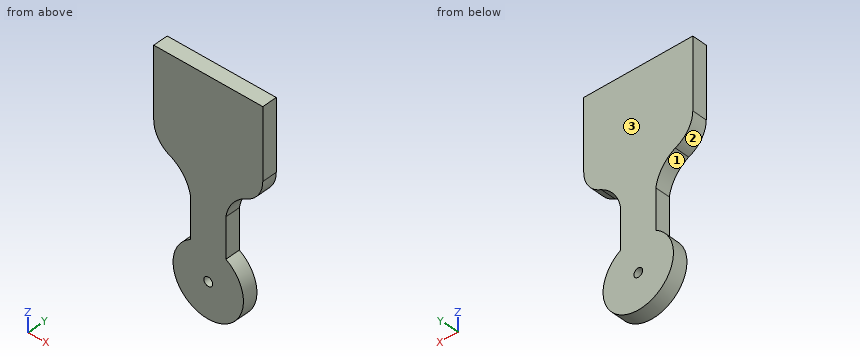
Autodesk Inventor part; units mm, degrees
ref_plane "YZ Plane" through (0, 0, 0) normal (1, 0, 0) x (0, 1, 0)
ref_plane "XZ Plane" through (0, 0, 0) normal (0, 1, 0) x (-1, 0, 0)
ref_plane "XY Plane" through (0, 0, 0) normal (0, 0, 1) x (1, 0, 0)
sketch "Sketch1" plane through (0, 0, 0) normal (0, 1, 0) x (-1, 0, 0)
  line L0 (-5, 10.0042) -> (5, 10.0042)
  line L1 (5, 10.0042) -> (5, -14.9958)
  line L2 (5, -14.9958) -> (-5, -14.9958)
  line L3 (-5, -14.9958) -> (-5, 10.0042)
  circle A0 centre (0, -24.9958) radius 10
  circle A1 centre (0, -24.9958) radius 1.25
  line L4 (-5, -14.9958) -> (-5, -16.3355)
  line L5 (5, -14.9958) -> (5, -16.3355)
  line L6 (-15.5, 30.0042) -> (15.5, 30.0042)
  line L7 (15.5, 30.0042) -> (15.5, 10.0042)
  line L8 (15.5, 10.0042) -> (-15.5, 10.0042)
  line L9 (-15.5, 10.0042) -> (-15.5, 30.0042)
  arc A2 (-5, -5) -> (-10.4985, 2.7374) centre (-15.4294, -6.5891) ccw
  arc A3 (-15.5, 10.0042) -> (-10.4985, 2.7374) centre (-7.7202, 10.0042) ccw
  line L10 (0, 46.7954) -> (0, -49.019) construction
  line L11 (-15.5, 10.0042) -> (-5, 10.0042)
  point P0 (0, 0)
  point P1 (0, -14.9958)
  point P2 (0, 10.0042)
  point P3 (0, 10.0042)
  dimension "d0" = 25
  dimension "d1" = 10
  dimension "d2" = 20
  dimension "d3" = 2.5
  dimension "d6" = 31
  dimension "d7" = 20
extrude "Extrusion1" add sketch "Sketch1" along normal blind 4.2 contours L8 L9 L6 L7 L0 | L0 L1 L2 L3 | L5 A0 L2 | L2 A0 L4 | A0
extrude "Extrusion2" add sketch "Sketch1" along normal blind 4.2 contours L3 A2 A3 L8
mirror "Mirror1" about plane through (0, 0, 0) normal (1, 0, 0) of "Extrusion2"
properties part number "ToolHolder"
Source: CAD feature listing. Evaluate the final solid. Frame: model axes, mm. Face numbers are marked on the shaded views. Coordinates: 2 decimals unless noted, no trailing zeros. Loops run counter-clockwise (first coordinate to the right, second up) from the corner with the lowest first, then second, coordinate; pieces in that order, holes last. Notation, with made-up numbers: (13.5, 39.5) -> (45.5, 39.5) arc R30 ccw to (45.5, 77.5) -> close; hole circle Ø9 at (81, 86.5). An arc over 180 degrees is marked (long way). One line per item, written item: value. Start each with the question number.
Q1. Line query: line 1 along Z through (x, y) = (0, 1.45); line 2 along Z through (x, y) = (-0.5, 3.4); line 3 along X through (y, z) = (0.35, -7). Output: solid intervals per line, ascending.
Q2. Section query B-B, the plane z = -7.5. Return the cut outline in (x, y), and give its area (3 significant figures).
Q3. Section query C-C, the plane x = 8. Return the cut outline in (y, z).
Q4. Contact query for flat-ended pins moving along their axis: P1, Ø1.5, axis at y = 1.5, z = -25, coming from the -X side; P2, Ø1.5, axis at x = 5, y = 1, coming from the -Z side; P3, Ø1.5, axis at y = 1.5, z = -7, coming from the -X side. Output: stop coordinate, or through.
Q5. Mould query, pull axis Z, two halves, no side actions, for the marked faces 1, 2 and 3. Classes: pulls with the +Z half, pulls with the -Z half, needs draft (parallel to the pull), parting line crosses it, or undercut.
Q6. Section query A-A, the plane x = 0. Return the cut outline in (y, z), and give its area (4 significant figures).
Results:
1. line 1: -35 to -26.25, -23.75 to 30
1. line 2: -34.98 to -26.14, -23.85 to 30
1. line 3: -5 to 5
2. outline: (-5, 0) -> (5, 0) -> (5, 4.2) -> (-5, 4.2) -> close
2. area: 42.0 mm^2
3. outline: (0, -31) -> (4.2, -31) -> (4.2, -19) -> (0, -19) -> close; (0, 0.9) -> (4.2, 0.9) -> (4.2, 30) -> (0, 30) -> close
4. P1: x = -10
4. P2: z = -34.05
4. P3: x = -5
5. face 1: undercut
5. face 2: pulls with the -Z half
5. face 3: needs draft
6. outline: (0, -35) -> (4.2, -35) -> (4.2, -26.25) -> (0, -26.25) -> close; (0, -23.75) -> (4.2, -23.75) -> (4.2, 30) -> (0, 30) -> close
6. area: 262.5 mm^2
